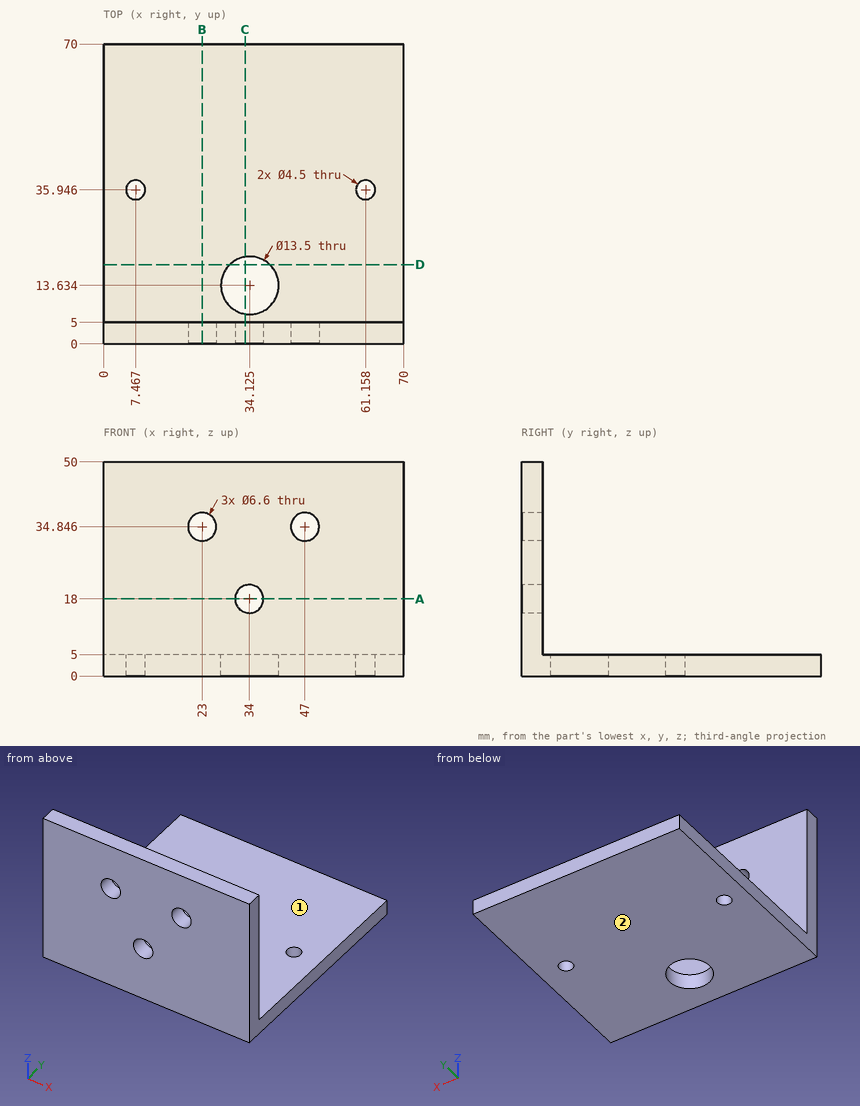
Can you work these out from the drawing? Everything is in mm from the part's minimum corner. A direction names the side the tool comes from. Round coordinates to 2 decimals unless told otherwise and drop trailing zeros. Order: outer loops, then holes, each group sorted by start corner. A loop starts at its lowest first (then second) coordinate and runs counter-clockwise, first axis right, second up.
(1) If we section it at A-A (z = 18): Please give me the cut outline in (x, y), plus the area to 3 significant figures.
Results are:
outline: (0, 0) - (30.7, 0) - (30.7, 5) - (0, 5) - close; (37.3, 0) - (70, 0) - (70, 5) - (37.3, 5) - close
area: 317 mm2
(2) If we section it at C-C (x = 33): Please give me the cut outline in (y, z) (1 decimal).
Results are:
outline: (0, 0) - (7, 0) - (7, 5) - (5, 5) - (5, 14.9) - (0, 14.9) - close; (0, 21.1) - (5, 21.1) - (5, 50) - (0, 50) - close; (20.3, 0) - (70, 0) - (70, 5) - (20.3, 5) - close
(3) I'm going to push flat-ended pins straight in: pin 1 (10.5 mm diameter, centred on x = 23, z = 34.85, fed in from +Y); pin 2 (7 mm diameter, centred on x = 7.47, y = 35.95, fed in from +Z). Where does each tip first touch, or does it pass through?
Results are:
pin 1: stops at y = 5
pin 2: stops at z = 5
(4) If we section it at D-D (y = 18.5): Please give me the cut outline in (x, z).
Results are:
outline: (0, 0) - (29.45, 0) - (29.45, 5) - (0, 5) - close; (38.8, 0) - (70, 0) - (70, 5) - (38.8, 5) - close
(5) On a 3-axis mill with a long thin cutter (end or side, diameter ignored), from which of +Z, -Z, +X, -X, +Y, -Y can I reach the whole of each face in a straight line? I mean the marked faces 1 and 2. Say none if no direction works.
Results are:
face 1: +Z, +X, -X, +Y
face 2: -Z, +X, -X, +Y, -Y
(6) If we section it at B-B (x = 23): Please give me the cut outline in (y, z) (1 decimal).
Results are:
outline: (0, 0) - (70, 0) - (70, 5) - (5, 5) - (5, 31.5) - (0, 31.5) - close; (0, 38.1) - (5, 38.1) - (5, 50) - (0, 50) - close
(7) If I drill on L1, parallel to Z at x = 23, y = 3.6 (1 decimal); L2, parallel to Y at x = 6, z = 27.5, over which ranges is the centre line in solid material (lowest first)?
Results are:
L1: z = 0 to 31.5, 38.1 to 50
L2: y = 0 to 5
